Part model, mm, in its own coordinate system. A direction names the side the tool comes from. Round coordinates to 2 decimals unless told otherwise and drop trailing zeros. Order: outer loops, then holes, each group sorted by start corner. A loop starts at its lowest first (then second) coordinate and runs counter-clockwise, first axis right, second up. Notation, with made-up numbers: (29.5, 28.25) -> (77.5, 28.25) arc R22 cw to (77.5, 56.25) -> close; hole circle Ø5 at (36.25, 60). An arc over 180 degrees is marked (long way). Return JSON: item names as keys, results as strings. Group by question number.
from build123d import *

# Parameters (mm, degrees)
F0_W     = 79.99999748
F0_H     = 64.99999954
F0_R     = 3.49999935
F1_DEPTH = 12.49999786
F2_D     = 11.99999886
F2_DEPTH = 3.49999808
F2_TIP   = 3.6051633717


with BuildPart() as f1:
    # F0 (on Top) → F1 (new body)
    with BuildSketch(Plane.XY):
        Rectangle(F0_W, F0_H)
        with Locations((-24.49999926, -22.49999818)):
            Circle(F0_R, mode=Mode.SUBTRACT)
        with Locations((24.49999926, -22.49999818)):
            Circle(F0_R, mode=Mode.SUBTRACT)
        with Locations((-24.49999926, 22.49999818)):
            Circle(F0_R, mode=Mode.SUBTRACT)
        with Locations((24.49999926, 22.49999818)):
            Circle(F0_R, mode=Mode.SUBTRACT)
    extrude(amount=-F1_DEPTH)

    # F2
    with Locations(Plane.XY):
        with Locations((24.49999926, -22.49999818), (-24.49999926, -22.49999818), (-24.49999926, 22.49999818), (24.49999926, 22.49999818)):
            Hole(F2_D / 2, depth=F2_DEPTH)
            with Locations((0, 0, -(F2_DEPTH + F2_TIP / 2))):  # 118° drill point
                Cone(0, F2_D / 2, F2_TIP, mode=Mode.SUBTRACT)


solid = f1.part
(1) Saw through at B-B, the plane x = -24.5. State how many separate pieces and enclosed holes the cut face has, and give its area (3 significant figures).
(2) Saw through at A-A, the plane z = -9.25. List the corners of the cut face in (x, y), and give its area (3 significant figures).
(3) Tool access for faces 1 (the flat face through (-1, 32.5, -6)), 2 (the cylindrical face through (21.274, -17.441, -1.774)): list every direction of +Z, -Z, +X, -X, +Y, -Y with a clear straight run to the whole face (end or side of a thin tool).
(4) Probe L1, parallel to Y at x = 24.5, z = -1.2; L2, parallel to Y at x = -24.5, z = -9.75; L3, parallel to X at y = 20, z = -3.25. List the from-to ranges inside material, lowest first. Write a range as [from, to].
(5) Mould opens along X. For faces 3 (the flat face through (-1, 0, -12.5)), 4 (the flat face through (-40, 0, -6)), 5 (the conical face through (23.71, 18.93, -4.91)) say: pulls with the +X half, pulls with the -X half, needs draft (parallel to the pull), parting line crosses it, or undercut.
(6) Pin check, flat tip, straight feed: P1, Ø6.5, axis at x = 24.5, y = 22.5, coming from the +Z side. Stop position of the tip, or through.
Results are:
{
 "1": {"separate pieces": "3", "enclosed holes": "0", "area": "595 mm^2"},
 "2": {"outline": "(-40, -32.5) -> (40, -32.5) -> (40, 32.5) -> (-40, 32.5) -> close; hole circle Ø7 at (-24.5, -22.5); hole circle Ø7 at (-24.5, 22.5); hole circle Ø7 at (24.5, -22.5); hole circle Ø7 at (24.5, 22.5)", "area": "5,050 mm^2"},
 "3": {"face 1": "+Z, -Z, +X, -X, +Y", "face 2": "+Z"},
 "4": {"L1": "y = [-32.5, -28.5], [-16.5, 16.5], [28.5, 32.5]", "L2": "y = [-32.5, -26], [-19, 19], [26, 32.5]", "L3": "x = [-40, -29.95], [-19.05, 19.05], [29.95, 40]"},
 "5": {"face 3": "needs draft", "face 4": "pulls with the -X half", "face 5": "undercut"},
 "6": {"P1": "passes through"}
}
